Model file for the job. Use its own axes, mm. Face numbers are marked on the shaded views. A direction names the side the tool comes from. Round coordinates to 2 decimals unless told otherwise and drop trailing zeros. Order: outer loops, then holes, each group sorted by start corner. A loop starts at its lowest first (then second) coordinate and runs counter-clockwise, first axis right, second up. Notation, with made-up numbers: (27.5, -13) - (74.5, -13) arc R31 ccw to (74.5, 19) - close; hole circle Ø4 at (73, -6). An arc over 180 degrees is marked (long way). Answer as CSV lines item,"result". Start each with the question number.
1. Band-saw the part on D-D on x = 26. List the corners of the cut face in (y, z) (3 decimals), then the cut area to 3 significant figures.
2. Band-saw the part on C-C on z = 35.5. List the corners of the cut face in (x, y) (3 decimals), then the cut area to 3 significant figures.
3. Wall check: line 1 along Y through (x, z) = (15, 33.5) (3 decimals); line 2 along Y through (x, z) = (0, 11). Give the ranges that are in metal, low to high. Write a range as [from, to].
4. Pull direction X, two halves, no side cores. Call the marked faces 1, 2 and 3: released by +X, released by -X, zero draft, split by the parting line, or undercut.
5. Band-saw the part on A-A on y = -8. List the corners of the cut face in (x, z) (3 decimals).
6. Band-saw the part on B-B on x = -35. List the corners of the cut face in (y, z) (3 decimals).
7. Pin check, flat tips, straight feed: pin 1 Ø5 at (x, y) = (-22, -12.5) entering from -Z; pin 2 Ø4 at (y, z) = (-38.5, 25) entering from -X; pin 3 Ø10 at (x, y) = (12.5, 33.5) entering from +Z; pin 4 Ø8 at (y, z) = (-38.5, 20) entering from +X. Stop position of each tip, or through.
8. 3-axis set-ups, long thin cutter, end or side, ignore diameter. For the marked faces 4 and 5: which of +Z, -Z, +X, -X, +Y, -Y reach the whole face in a straight line?
```python
from build123d import *

# Parameters (mm, degrees)
SKETCH_1_R          = 5
SKETCH_1_R_2        = 42.84145639
EXTRUDE_2_DEPTH     = 40
SKETCH_1_5_R        = 42.84145639
EXTRUDE_3_DEPTH     = 5
CUT_EXTRUDE_START   = 25
CUT_EXTRUDE_2_DEPTH = 25
SKETCH_5_R          = 30
SKETCH_5_R_2        = 2.5
CUT_EXTRUDE_3_DEPTH = 82.240384046
CUT_EXTRUDE_4_DEPTH = 10


with BuildPart() as part:
    # Sketch 1 → Extrude 2 (new body)
    with BuildSketch(Plane.XY):
        with BuildLine():
            Line((-30.293484329, 50), (30.293484329, 50))
            ThreePointArc((30.293484329, 50), (44.228095194, 44.228095194), (50, 30.293484329))
            Line((50, 30.293484329), (50, -30.293484329))
            ThreePointArc((50, -30.293484329), (44.228095194, -44.228095194), (30.293484329, -50))
            Line((30.293484329, -50), (-30.293484329, -50))
            ThreePointArc((-30.293484329, -50), (-44.228095194, -44.228095194), (-50, -30.293484329))
            Line((-50, -30.293484329), (-50, 30.293484329))
            ThreePointArc((-50, 30.293484329), (-44.228095194, 44.228095194), (-30.293484329, 50))
        make_face()
        with Locations((-38.635004029, 38.635004029)):
            Circle(SKETCH_1_R, mode=Mode.SUBTRACT)
        with Locations(Location((38.635004029, 38.635004029, 0), (0, 0, 180))):
            Circle(SKETCH_1_R, mode=Mode.SUBTRACT)
        with Locations((38.635004029, -38.635004029)):
            Circle(SKETCH_1_R, mode=Mode.SUBTRACT)
        with Locations(Location((-38.635004029, -38.635004029, 0), (0, 0, 180))):
            Circle(SKETCH_1_R, mode=Mode.SUBTRACT)
        Circle(SKETCH_1_R_2, mode=Mode.SUBTRACT)
    extrude(amount=EXTRUDE_2_DEPTH)

    # Sketch 1_5 → Extrude 3 (add)
    with BuildSketch(Plane.XY):
        Circle(SKETCH_1_5_R)
    extrude(amount=EXTRUDE_3_DEPTH)

    # Sketch 4 → Cut-Extrude 2 (cut)
    with BuildSketch(Plane(origin=(0, 0, 40), x_dir=(-1, 0, 0), z_dir=(0, 0, -1)).offset(CUT_EXTRUDE_START)):
        with BuildLine():
            Line((-38.635004029, 43.635004029), (38.635004029, 43.635004029))
            ThreePointArc((38.635004029, 43.635004029), (42.170537935, 42.170537935), (43.635004029, 38.635004029))
            Line((43.635004029, 38.635004029), (43.635004029, -38.635004029))
            ThreePointArc((43.635004029, -38.635004029), (42.170537935, -42.170537935), (38.635004029, -43.635004029))
            Line((38.635004029, -43.635004029), (-38.635004029, -43.635004029))
            ThreePointArc((-38.635004029, -43.635004029), (-42.170537935, -42.170537935), (-43.635004029, -38.635004029))
            Line((-43.635004029, -38.635004029), (-43.635004029, 38.635004029))
            ThreePointArc((-43.635004029, 38.635004029), (-42.170537935, 42.170537935), (-38.635004029, 43.635004029))
        make_face()
    extrude(amount=-CUT_EXTRUDE_2_DEPTH, mode=Mode.SUBTRACT)

    # Sketch 5 → Cut-Extrude 3 (cut, through all)
    with BuildSketch(Plane(origin=(0, 0, 0), x_dir=(-1, 0, 0), z_dir=(0, 0, -1))):
        with Locations((0.201090543, 0.15997854)):
            Circle(SKETCH_5_R)
        with Locations((-24.798909457, 25.15997854)):
            Circle(SKETCH_5_R_2)
        with Locations(Location((25.201090543, 25.15997854, 0), (0, 0, 180))):
            Circle(SKETCH_5_R_2)
        with Locations((25.201090543, -24.84002146)):
            Circle(SKETCH_5_R_2)
        with Locations(Location((-25.201090543, -24.84002146, 0), (0, 0, 180))):
            Circle(SKETCH_5_R_2)
    extrude(amount=-CUT_EXTRUDE_3_DEPTH, mode=Mode.SUBTRACT)

    # Sketch 7 → Cut-Extrude 4 (cut)
    with BuildSketch(Plane.ZY.offset(50)):
        with BuildLine():
            Line((29, 14), (29, -14))
            ThreePointArc((29, -14), (23, -20), (17, -14))
            Line((17, -14), (17, 14))
            ThreePointArc((17, 14), (23, 20), (29, 14))
        make_face()
    cut_extrude_4 = extrude(amount=-CUT_EXTRUDE_4_DEPTH, mode=Mode.SUBTRACT)

    # Mirror 1: Cut-Extrude 4 across plane
    add(cut_extrude_4.mirror(Plane(origin=(0, 0, 0), x_dir=(0, 0, 1), z_dir=(1, 0, 0))), mode=Mode.SUBTRACT)

    # Mirror 2: Cut-Extrude 4 across plane
    add(cut_extrude_4.mirror(Plane(origin=(0, 0, 0), x_dir=(0, 0, 1), z_dir=(0.7071067811865475, 0.7071067811865477, 0))), mode=Mode.SUBTRACT)


solid = part.part
```
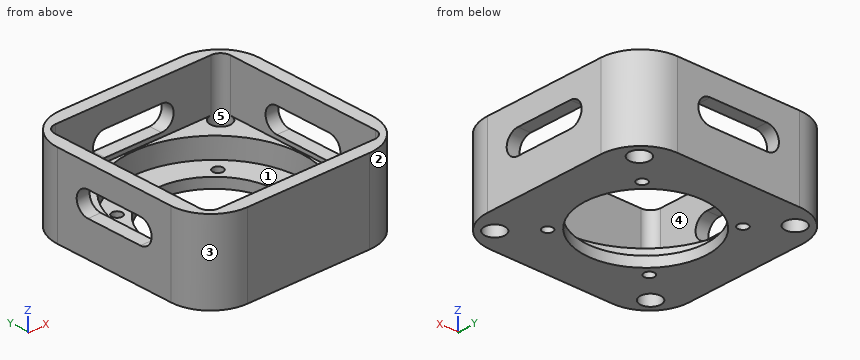
Reply:
1,outline,"(-50, 0) - (-27.209, 0) - (-27.209, 5) - (-34.05, 5) - (-34.05, 15) - (-43.635, 15) - (-43.635, 40) - (-50, 40) - close; (-22.471, 0) - (-14.452, 0) - (-14.452, 5) - (-22.471, 5) - close; (14.772, 0) - (22.967, 0) - (22.967, 5) - (14.772, 5) - close; (27.353, 0) - (50, 0) - (50, 40) - (43.635, 40) - (43.635, 15) - (34.05, 15) - (34.05, 5) - (27.353, 5) - close"
1,area,"946 mm2"
2,outline,"(-50, -30.293) arc R19.707 ccw to (-30.293, -50) - (30.293, -50) arc R19.707 ccw to (50, -30.293) - (50, 30.293) arc R19.707 ccw to (30.293, 50) - (-30.293, 50) arc R19.707 ccw to (-50, 30.293) - close; hole (-43.635, -38.635) arc R5 ccw to (-38.635, -43.635) - (38.635, -43.635) arc R5 ccw to (43.635, -38.635) - (43.635, 38.635) arc R5 ccw to (38.635, 43.635) - (-38.635, 43.635) arc R5 ccw to (-43.635, 38.635) - close"
2,area,"2,070 mm2"
3,line 1,"y = [-50, -43.635], [43.635, 50]"
3,line 2,"y = [-50, -42.84], [42.84, 50]"
4,face 1,"undercut"
4,face 2,"released by +X"
4,face 3,"released by -X"
5,outline,"(-50, 0) - (-29.07, 0) - (-29.07, 5) - (-42.088, 5) - (-42.088, 15) - (-43.635, 15) - (-43.635, 17) - (-50, 17) - close; (-50, 29) - (-43.635, 29) - (-43.635, 40) - (-50, 40) - close; (28.668, 0) - (50, 0) - (50, 17) - (43.635, 17) - (43.635, 15) - (42.088, 15) - (42.088, 5) - (28.668, 5) - close; (43.635, 29) - (50, 29) - (50, 40) - (43.635, 40) - close"
6,outline,"(-49.43, 0) - (-42.068, 0) - (-42.068, 15) - (-43.635, 15) - (-43.635, 40) - (-49.43, 40) - close; (-35.202, 0) - (35.202, 0) - (35.202, 15) - (24.706, 15) - (24.706, 5) - (-24.706, 5) - (-24.706, 15) - (-35.202, 15) - close; (42.068, 0) - (49.43, 0) - (49.43, 40) - (43.635, 40) - (43.635, 15) - (42.068, 15) - close"
7,pin 1,"passes through"
7,pin 2,"stops at x = -49"
7,pin 3,"stops at z = 5"
7,pin 4,"stops at x = 49.55"
8,face 4,"+Z"
8,face 5,"+Z, -Z"
